from build123d import *

# Parameters (mm, degrees)
F0_R     = 8
F1_DEPTH = 2.5
F2_R     = 7
F3_DEPTH = 0.5
F4_R     = 3.5
F5_DEPTH = 0.5
F6_R     = 2.5
F7_DEPTH = 25
F9_SIZE  = 0.3


with BuildPart() as f1:
    # F0 (on Top) → F1 (new body)
    with BuildSketch(Plane.XY):
        Circle(F0_R)
    extrude(amount=F1_DEPTH)

    # F2 (on face) → F3 (cut)
    with BuildSketch(Plane.XY.offset(2.5)):
        Circle(F2_R)
    extrude(amount=-F3_DEPTH, mode=Mode.SUBTRACT)

    # F4 (on face) → F5 (join)
    with BuildSketch(Plane.XY.offset(2)):
        Circle(F4_R)
    extrude(amount=F5_DEPTH)

    # F6 (on face) → F7 (cut)
    with BuildSketch(Plane.XY.offset(2.5)):
        Circle(F6_R)
    extrude(amount=-F7_DEPTH, mode=Mode.SUBTRACT)

    # F8: F1 across face


with BuildPart() as f1_1:
    add(f1.part)
    add(f1.part.mirror(Plane(origin=(0, 0, 0), x_dir=(1, 0, 0), z_dir=(0, 0, -1))))

    # F9
    f9_edges = [f1_1.edges().sort_by_distance(p)[0] for p in [
        (-8, 0, 2.5),
        (-8, 0, -2.5),
    ]]
    chamfer(f9_edges, length=F9_SIZE)


solid = f1_1.part
Geometry: final body of the model. Coordinates: model frame, mm. A direction names the side the tool comes from. Coordinates: 2 decimals unless noted, no trailing zeros. Order: outer loops, then holes, each group sorted by start corner. A loop starts at its lowest first (then second) coordinate and runs counter-clockwise, first axis right, second up.
1) Section C-C (z = 1.2). Return loops of the section in (x, y).
Result sheet:
outline: circle Ø16 at (0, 0); hole circle Ø5 at (0, 0)
2) First-contact query: P1, Ø3, axis at x = 4.5, z = 1, coming from the -Y side; P2, Ø1, axis at x = 4, z = 1, coming from the -Y side; P3, Ø6.5, axis at x = 0, y = 0, coming from the +Z side; P4, Ø2, axis at x = 1, y = -5, coming from the -Z side. Flat tips, straight axial feed; report the tip coordinate or a pass-through.
Result sheet:
P1: stops at y = -7.42
P2: stops at y = -7.19
P3: stops at z = 2.5
P4: stops at z = -2
3) Ray query, probe 1 along Y at (x, z) = (0, -0.6); probe 2 along Z at (x, y) = (2.25, 4); probe 3 along X at (y, z) = (1, -0.75). Return the intervals inside material, ascending.
Result sheet:
probe 1: y = -8 to -2.5, 2.5 to 8
probe 2: z = -2 to 2
probe 3: x = -7.94 to -2.29, 2.29 to 7.94
4) Set-up query: faces 1 (the cylindrical face through (6.466, -2.681, 2.254)), 2 (the flat face through (3, -3, -2)), 3 (the flat face through (2, -2, 2.5)). Return all of +Z, -Z, +X, -X, +Y, -Y with unobstructed straight access to the full face (end or side cutting, diameter ignored); none if empty.
Result sheet:
face 1: +Z
face 2: -Z
face 3: +Z, +X, -X, +Y, -Y
5) Draft query along Y for faces 4 (the cylindrical face through (3.233, -1.341, -2.246)), 5 (the cylindrical face through (-1.73, -7.81, 0.03)), 6 (the flat face through (2, -7, 2.5)). Return one class per face: released by +Y, released by -Y, zero draft, split by the parting line, or undercut.
Result sheet:
face 4: undercut
face 5: split by the parting line
face 6: zero draft
6) Section A-A (x = 0). Return loops of the section in (y, z), then the cut area to 3 significant figures.
Result sheet:
outline: (-8, -2.2) - (-7.7, -2.5) - (-7, -2.5) - (-7, -2) - (-3.5, -2) - (-3.5, -2.5) - (-2.5, -2.5) - (-2.5, 2.5) - (-3.5, 2.5) - (-3.5, 2) - (-7, 2) - (-7, 2.5) - (-7.7, 2.5) - (-8, 2.2) - close; (2.5, -2.5) - (3.5, -2.5) - (3.5, -2) - (7, -2) - (7, -2.5) - (7.7, -2.5) - (8, -2.2) - (8, 2.2) - (7.7, 2.5) - (7, 2.5) - (7, 2) - (3.5, 2) - (3.5, 2.5) - (2.5, 2.5) - close
area: 47.8 mm2
